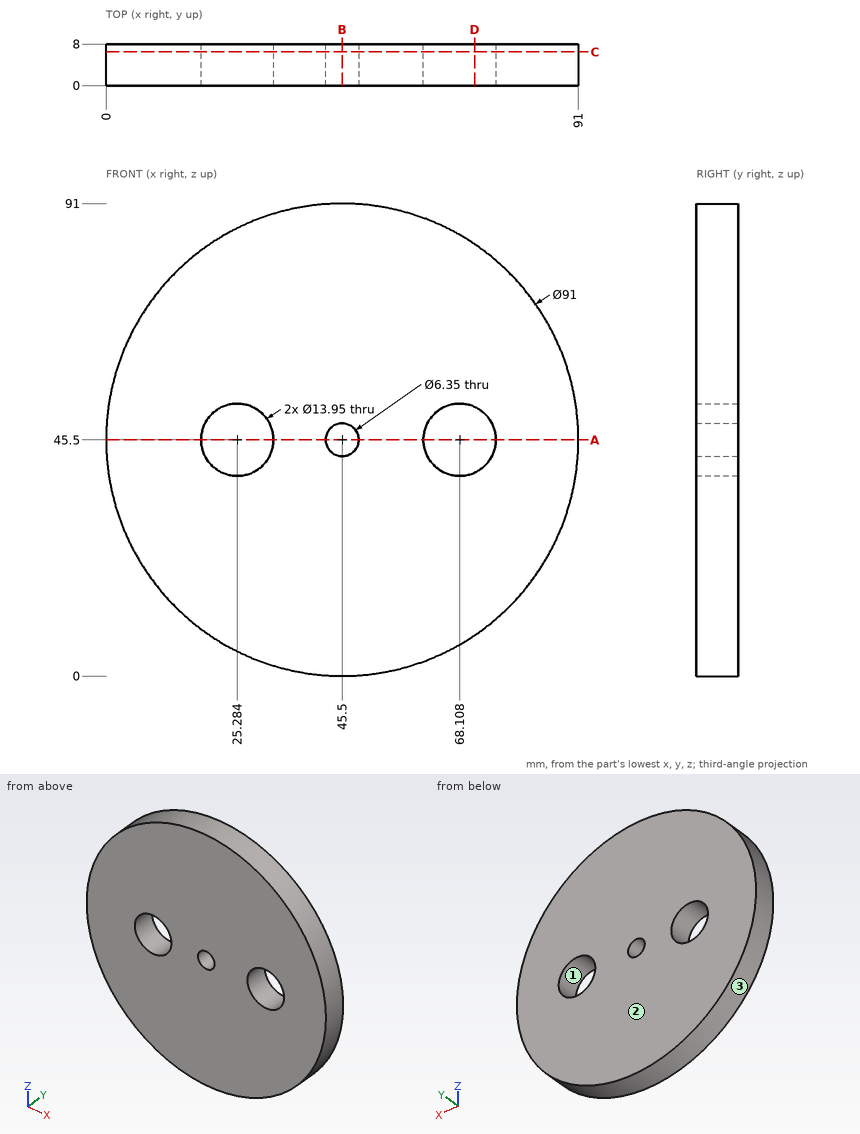
Can you work these out from the drawing? Everything is in mm from the part's minimum corner. Round coordinates to 2 decimals unless told otherwise and drop trailing zeros. Write each loop counter-clockwise with the first axis right and the second up, starting at its lowest first coordinate (ties: lowest second). Pieces come first, ordered by that corner, then holes. Notation, with made-up numbers: (83, 82) - (118, 82) arc R7 ccw to (118, 91) - close; hole circle Ø7 at (21.25, 66.25). An arc over 180 degrees is marked (long way). Use a Markdown table: item, result.
Q1. Thinking about a two-plate mould opening in X: for the marked faces 1, 2 and 3, which applies, released by +X, released by -X, zero draft, split by the parting line, or undercut?
Output values:
| item | result |
|---|---|
| face 1 | undercut |
| face 2 | zero draft |
| face 3 | split by the parting line |
Q2. I want a section at B-B (x = 45.5). List the corners of the cut face in (y, z) for me (3 decimals), plus the area to 3 significant figures.
Output values:
| item | result |
|---|---|
| outline | (0, 0) - (8, 0) - (8, 42.325) - (0, 42.325) - close; (0, 48.675) - (8, 48.675) - (8, 91) - (0, 91) - close |
| area | 677 mm2 |
Q3. I want a section at D-D (x = 71). List the corners of the cut face in (y, z) for me.
Output values:
| item | result |
|---|---|
| outline | (0, 7.82) - (8, 7.82) - (8, 39.15) - (0, 39.15) - close; (0, 51.85) - (8, 51.85) - (8, 83.18) - (0, 83.18) - close |
Q4. For pin 1 (3 mm diameter, centred on x = 36, y = 6, fed in from +Z); pin 2 (1 mm diameter, centred on x = 72, y = 3.5, fed in from -Z); pin 3 (1.5 mm diameter, centred on x = 16, y = 6.5, fed in from +Z), each with a flat end and sliding along its axis, tell me the tip position at first contact or that it passes through.
Output values:
| item | result |
|---|---|
| pin 1 | z = 90.29 |
| pin 2 | z = 8.16 |
| pin 3 | z = 80.77 |
Q5. I want a section at A-A (z = 45.5). List the corners of the cut face in (x, y) for me (1 decimal), plus the area to 3 significant figures.
Output values:
| item | result |
|---|---|
| outline | (0, 0) - (18.3, 0) - (18.3, 8) - (0, 8) - close; (32.3, 0) - (42.3, 0) - (42.3, 8) - (32.3, 8) - close; (48.7, 0) - (61.1, 0) - (61.1, 8) - (48.7, 8) - close; (75.1, 0) - (91, 0) - (91, 8) - (75.1, 8) - close |
| area | 454 mm2 |
Q6. I want a section at C-C (y = 6.5). Count the separate pieces of the cut face and the enclosed holes in it, plus the area to 3 significant figures.
Output values:
| item | result |
|---|---|
| separate pieces | 1 |
| enclosed holes | 3 |
| area | 6,170 mm2 |
Q7. Please list where these lines run through material, in increasing order: L1, parallel to X at y = 7.5, z = 44.5 (1 decimal); L2, parallel to Z at x = 26.5, y = 5.25; L3, parallel to Z at x = 79, y = 5.5.
Output values:
| item | result |
|---|---|
| L1 | 0 to 18.4, 32.2 to 42.5, 48.5 to 61.2, 75 to 91 |
| L2 | 4.16 to 38.63, 52.37 to 86.84 |
| L3 | 14.71 to 76.29 |
